Geometry check sheet. Reference: drawing and pictorial views, mm from the part's lowest x, y, z. A direction names the side the tool comes from. Give positions to 0.01 mm unless a question says otherwise; leave off trailing zeros. Write each loop counter-clockwise with the first axis right and the second up, starting at its lowest first coordinate (ties: lowest second). Pieces come first, ordered by that corner, then holes. Notation, with made-up numbers: M 64,1.5 L 71,1.5 A17 cw 71,15.5 Z; hole C 69.25,55.5 d8. An arc over 180 degrees is marked long. One line per item, written item: value. Start each with the question number.
1. Scan lines: line 1 (Y direction, x = 18.75, z = 9.5); line 2 (X direction, y = 13.5, z = 6.75); line 3 (Z direction, x = 3.25, y = 18.5). Record each from-to range of solid material in increasing order.
2. Cross-section at C-C on x = 16.25. Record the cut outline in (y, z).
3. Cross-section at B-B on y = 7.5. Record the cut outline in (x, z).
4. Cross-section at A-A on z = 4. Record the cut outline in (x, y).
5. Tool access check on the marked faces 1, 2 and 3. Record the directions out of +Z, -Z, +X, -X, +Y, -Y that give a thin tool (end or side, any length) a straight path to the whole face; none if there is none.
6. Release check for a two-part mould opening along X. For the marked faces 4, 5 and 6 record: pulls with the +X half, pulls with the -X half, needs draft (parallel to the pull), parting line crosses it, or undercut.
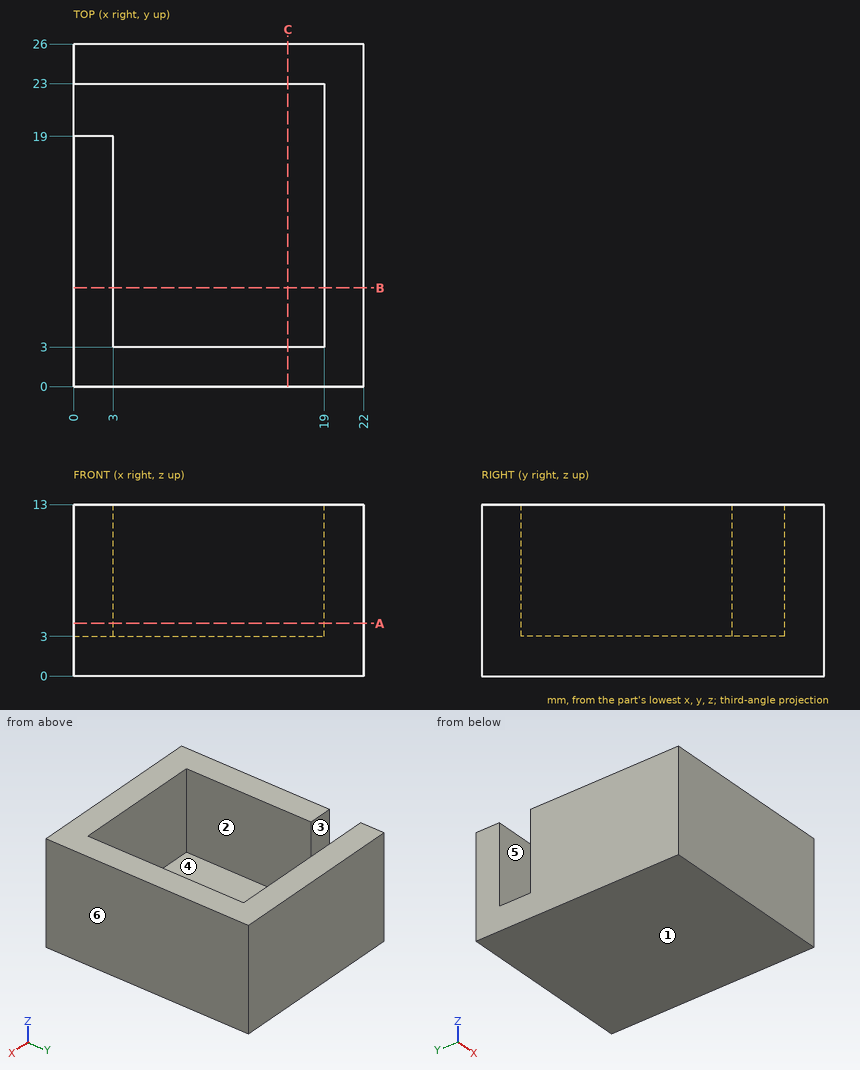
Report:
1. line 1: y = 0 to 3, 23 to 26
1. line 2: x = 0 to 3, 19 to 22
1. line 3: z = 0 to 3
2. outline: M 0,0 L 26,0 L 26,13 L 23,13 L 23,3 L 3,3 L 3,13 L 0,13 Z
3. outline: M 0,0 L 22,0 L 22,13 L 19,13 L 19,3 L 3,3 L 3,13 L 0,13 Z
4. outline: M 0,0 L 22,0 L 22,26 L 0,26 L 0,23 L 19,23 L 19,3 L 3,3 L 3,19 L 0,19 Z
5. face 1: -Z, +X, -X, +Y, -Y
5. face 2: +Z
5. face 3: +Z, -X
6. face 4: undercut
6. face 5: needs draft
6. face 6: pulls with the +X half
